Check sheet for the modelled part. Datum: model origin and axes. Units: mm. A direction names the side the tool comes from. Coordinates: 2 decimals unless noted, no trailing zeros. Write each loop counter-clockwise with the first axis right and the second up, starting at its lowest first coordinate (ties: lowest second). Pieces come first, ordered by that corner, then holes. Notation, with made-up numbers: (39.5, -9.75) - (86.5, -9.75) arc R16 ccw to (86.5, 9.25) - close; hole circle Ø11 at (42.5, 34.25). An arc over 180 degrees is marked (long way). Use one line per item in the form item = value. Start each with the question number.
1. Cross-section at B-B on y = -3.75. Record the boundary of the cut face in (x, z).
2. Cross-section at D-D on y = -8. Record the boundary of the cut face in (x, z), then the cut area to 3 significant figures.
3. Cross-section at C-C on x = 14.5. Record the boundary of the cut face in (y, z), then the cut area to 3 significant figures.
4. Draft check along Y on faces 1 (the face through (-6, -13, 18.043)), 2 (the face through (-4, -15, 23)), 3 (the face through (4, 10.05, 2)), 4 (the face through (-35, 5.95, 42)). Enter one of: +Y half, -Y half, draft (parallel to the pull), parting line (faces both ways), or undercut.
5. Tool access check on faces 5 (the face through (-13.007, -13.479, 19.751)), 6 (the face through (29, -2, 2)), 7 (the face through (-34.96, 8.05, 63.55)), 8 (the face through (4, -5.95, 2)). Record the directions out of +Z, -Z, +X, -X, +Y, -Y that give a thin tool (end or side, any length) a straight path to the whole face; none if there is none.
6. Go/stop test with flat-tipped pins: pin 1 Ø5.5 at (x, z) = (-17, 33) entering from +Y; pin 2 Ø3.5 at (x, z) = (-15.5, 20) entering from +Y; pin 3 Ø0.9 at (x, y) = (-5.5, -14) entering from +Z; pin 4 Ø3.5 at (x, z) = (-15.99, 41.51) entering from -Y. Record where each tip stops, or that it passes through.
7. Scan lines: line 1 along Z through (x, y) = (-15.5, -12.25); line 2 along X through (y, z) = (3, 58.5); line 3 along Y through (x, z) = (-30, 41.5). Record each from-to range of solid material in increasing order.
8. Cross-section at A-A on z = 46.5. Record the boundary of the cut face in (x, y), then the cut area to 4 significant figures.
```python
from build123d import *

# Parameters (mm, degrees)
F1_DEPTH = 5
F3_ANGLE = 90
F7_R     = 2.05
F8_DEPTH = 5
F9_DEPTH = 3


# Not quite as in the source:
# - a feature names something its author has since deleted; it is built from what else it names


with BuildPart() as f1:
    # F0 (on Top) → F1 (new body)
    with BuildSketch(Plane.XY):
        Polygon((29, 12), (-21, 12), (-21, -12), (0, -12), (29, -12), align=None)
        with BuildLine():
            ThreePointArc((-16, -10.05), (-18.05, -8), (-16, -5.95))
            Line((-16, -5.95), (0, -5.95))
            Line((0, -5.95), (24, -5.95))
            ThreePointArc((24, -5.95), (26.05, -8), (24, -10.05))
            Line((24, -10.05), (0, -10.05))
            Line((0, -10.05), (-16, -10.05))
        make_face(mode=Mode.SUBTRACT)
        with BuildLine():
            Line((0, -2.05), (-16, -2.05))
            ThreePointArc((-16, -2.05), (-18.05, 0), (-16, 2.05))
            Line((-16, 2.05), (0, 2.05))
            Line((0, 2.05), (24, 2.05))
            ThreePointArc((24, 2.05), (26.05, 0), (24, -2.05))
            Line((24, -2.05), (0, -2.05))
        make_face(mode=Mode.SUBTRACT)
        with BuildLine():
            Line((24, 5.95), (0, 5.95))
            Line((0, 5.95), (-16, 5.95))
            ThreePointArc((-16, 5.95), (-18.05, 8), (-16, 10.05))
            Line((-16, 10.05), (0, 10.05))
            Line((0, 10.05), (24, 10.05))
            ThreePointArc((24, 10.05), (26.05, 8), (24, 5.95))
        make_face(mode=Mode.SUBTRACT)
    extrude(amount=F1_DEPTH)


with BuildPart() as f3_1:
    # F3: copy of F1
    add(f1.part.rotate(Axis((-21, 0, 2.5), (0, -1, 0)), F3_ANGLE))


with BuildPart() as f3_1_1:
    # F4: moved
    add(f3_1.part.moved(Location((0, 0, 14))))


with BuildPart() as f3_1_2:
    # F5: moved
    add(f3_1_1.part.moved(Location((-14, 0, 0))))


with BuildPart() as f1_1:
    add(f1.part)

    add(f3_1_2.part)  # F8 merges F3_1
    # F7 (on 3pt) → F8 (join)
    with BuildSketch(Plane.XZ.offset(12)):
        Polygon((-37.5, 16.5), (-21, 0), (29, 0), (29, 5), (-32.5, 66.5), (-37.5, 66.5), align=None)
        Polygon((-19.9926406871, 21.5073593129), (-17.9926406871, 24.971460928), (-13.9926406871, 24.971460928), (-11.9926406871, 21.5073593129), (-13.9926406871, 18.0432576977), (-17.9926406871, 18.0432576977), align=None, mode=Mode.SUBTRACT)
        Polygon((-9.9926406871, 21.5073593129), (-7.9926406871, 24.971460928), (-3.9926406871, 24.971460928), (-1.9926406871, 21.5073593129), (-3.9926406871, 18.0432576977), (-7.9926406871, 18.0432576977), align=None, mode=Mode.SUBTRACT)
        Polygon((-19.9926406871, 31.5073593129), (-17.9926406871, 34.971460928), (-13.9926406871, 34.971460928), (-11.9926406871, 31.5073593129), (-13.9926406871, 28.0432576977), (-17.9926406871, 28.0432576977), align=None, mode=Mode.SUBTRACT)
        Polygon((-9.8563439923, 30.4720831325), (-8.8210678119, 34.3357864376), (-4.9573645067, 35.371062618), (-2.128937382, 32.5426354933), (-3.1642135624, 28.6789321881), (-7.0279168675, 27.6436560077), align=None, mode=Mode.SUBTRACT)
        Polygon((0.1436560077, 20.4720831325), (1.1789321881, 24.3357864376), (5.0426354933, 25.371062618), (7.871062618, 22.5426354933), (6.8357864376, 18.6789321881), (2.9720831325, 17.6436560077), align=None, mode=Mode.SUBTRACT)
        Polygon((-19.8563439923, 40.4720831325), (-18.8210678119, 44.3357864376), (-14.9573645067, 45.371062618), (-12.128937382, 42.5426354933), (-13.1642135624, 38.6789321881), (-17.0279168675, 37.6436560077), align=None, mode=Mode.SUBTRACT)
        Polygon((-4.9573645067, 35.371062618), (-8.8210678119, 34.3357864376), (-9.8563439923, 30.4720831325), (-7.0279168675, 27.6436560077), (-3.1642135624, 28.6789321881), (-2.128937382, 32.5426354933), align=None)
        with Locations((-5.9926406871, 31.5073593129)):
            Circle(F7_R, mode=Mode.SUBTRACT)
        Polygon((-14.9573645067, 45.371062618), (-18.8210678119, 44.3357864376), (-19.8563439923, 40.4720831325), (-17.0279168675, 37.6436560077), (-13.1642135624, 38.6789321881), (-12.128937382, 42.5426354933), align=None)
        with Locations((-15.9926406871, 41.5073593129)):
            Circle(F7_R, mode=Mode.SUBTRACT)
        Polygon((-13.9926406871, 34.971460928), (-17.9926406871, 34.971460928), (-19.9926406871, 31.5073593129), (-17.9926406871, 28.0432576977), (-13.9926406871, 28.0432576977), (-11.9926406871, 31.5073593129), align=None)
        with Locations((-15.9926406871, 31.5073593129)):
            Circle(F7_R, mode=Mode.SUBTRACT)
        Polygon((-13.9926406871, 24.971460928), (-17.9926406871, 24.971460928), (-19.9926406871, 21.5073593129), (-17.9926406871, 18.0432576977), (-13.9926406871, 18.0432576977), (-11.9926406871, 21.5073593129), align=None)
        with Locations((-15.9926406871, 21.5073593129)):
            Circle(F7_R, mode=Mode.SUBTRACT)
        Polygon((-3.9926406871, 24.971460928), (-7.9926406871, 24.971460928), (-9.9926406871, 21.5073593129), (-7.9926406871, 18.0432576977), (-3.9926406871, 18.0432576977), (-1.9926406871, 21.5073593129), align=None)
        with Locations((-5.9926406871, 21.5073593129)):
            Circle(F7_R, mode=Mode.SUBTRACT)
        Polygon((5.0426354933, 25.371062618), (1.1789321881, 24.3357864376), (0.1436560077, 20.4720831325), (2.9720831325, 17.6436560077), (6.8357864376, 18.6789321881), (7.871062618, 22.5426354933), align=None)
        with Locations((4.0073593129, 21.5073593129)):
            Circle(F7_R, mode=Mode.SUBTRACT)
    extrude(amount=F8_DEPTH)

    # F7 (on 3pt) → F9 (cut)
    with BuildSketch(Plane.XZ.offset(12)):
        Polygon((-4.9573645067, 35.371062618), (-8.8210678119, 34.3357864376), (-9.8563439923, 30.4720831325), (-7.0279168675, 27.6436560077), (-3.1642135624, 28.6789321881), (-2.128937382, 32.5426354933), align=None)
        with Locations((-5.9926406871, 31.5073593129)):
            Circle(F7_R, mode=Mode.SUBTRACT)
        Polygon((5.0426354933, 25.371062618), (1.1789321881, 24.3357864376), (0.1436560077, 20.4720831325), (2.9720831325, 17.6436560077), (6.8357864376, 18.6789321881), (7.871062618, 22.5426354933), align=None)
        with Locations((4.0073593129, 21.5073593129)):
            Circle(F7_R, mode=Mode.SUBTRACT)
        Polygon((-3.9926406871, 24.971460928), (-7.9926406871, 24.971460928), (-9.9926406871, 21.5073593129), (-7.9926406871, 18.0432576977), (-3.9926406871, 18.0432576977), (-1.9926406871, 21.5073593129), align=None)
        with Locations((-5.9926406871, 21.5073593129)):
            Circle(F7_R, mode=Mode.SUBTRACT)
        Polygon((-13.9926406871, 24.971460928), (-17.9926406871, 24.971460928), (-19.9926406871, 21.5073593129), (-17.9926406871, 18.0432576977), (-13.9926406871, 18.0432576977), (-11.9926406871, 21.5073593129), align=None)
        with Locations((-15.9926406871, 21.5073593129)):
            Circle(F7_R, mode=Mode.SUBTRACT)
        Polygon((-13.9926406871, 34.971460928), (-17.9926406871, 34.971460928), (-19.9926406871, 31.5073593129), (-17.9926406871, 28.0432576977), (-13.9926406871, 28.0432576977), (-11.9926406871, 31.5073593129), align=None)
        with Locations((-15.9926406871, 31.5073593129)):
            Circle(F7_R, mode=Mode.SUBTRACT)
        Polygon((-14.9573645067, 45.371062618), (-18.8210678119, 44.3357864376), (-19.8563439923, 40.4720831325), (-17.0279168675, 37.6436560077), (-13.1642135624, 38.6789321881), (-12.128937382, 42.5426354933), align=None)
        with Locations((-15.9926406871, 41.5073593129)):
            Circle(F7_R, mode=Mode.SUBTRACT)
    extrude(amount=F9_DEPTH, mode=Mode.SUBTRACT)


solid = f1_1.part
```
Final values:
q1.outline = (-37.5, 16.5) - (-32.5, 16.5) - (-32.5, 66.5) - (-37.5, 66.5) - close; (-21, 0) - (29, 0) - (29, 5) - (-21, 5) - close
q2.outline = (-37.5, 16.5) - (-32.5, 16.5) - (-32.5, 19.45) - (-37.5, 19.45) - close; (-37.5, 63.55) - (-32.5, 63.55) - (-32.5, 66.5) - (-37.5, 66.5) - close; (-21, 0) - (-18.05, 0) - (-18.05, 5) - (-21, 5) - close; (26.05, 0) - (29, 0) - (29, 5) - (26.05, 5) - close
q2.area = 59.0 mm²
q3.outline = (-17, 0) - (-10.05, 0) - (-10.05, 5) - (-12, 5) - (-12, 19.5) - (-17, 19.5) - close; (-5.95, 0) - (-2.05, 0) - (-2.05, 5) - (-5.95, 5) - close; (2.05, 0) - (5.95, 0) - (5.95, 5) - (2.05, 5) - close; (10.05, 0) - (12, 0) - (12, 5) - (10.05, 5) - close
q3.area = 156 mm²
q4.face_1 = draft
q4.face_2 = +Y half
q4.face_3 = undercut
q4.face_4 = undercut
q5.face_5 = +Y
q5.face_6 = +Z, -Z, +X, +Y, -Y
q5.face_7 = +X, -X
q5.face_8 = +Z, -Z
q6.pin_1 = -12
q6.pin_2 = -15
q6.pin_3 = 39.95
q6.pin_4 = through
q7.line_1 = 0 to 18.04, 24.97 to 28.04, 34.97 to 38.05, 45.23 to 49.5
q7.line_2 = -37.5 to -32.5
q7.line_3 = -17 to -12
q8.outline = (-37.5, -17) - (-12.5, -17) - (-12.5, -12) - (-32.5, -12) - (-32.5, -10.05) - (-37.5, -10.05) - close; (-37.5, -5.95) - (-32.5, -5.95) - (-32.5, -2.05) - (-37.5, -2.05) - close; (-37.5, 2.05) - (-32.5, 2.05) - (-32.5, 5.95) - (-37.5, 5.95) - close; (-37.5, 10.05) - (-32.5, 10.05) - (-32.5, 12) - (-37.5, 12) - close
q8.area = 183.5 mm²
